Geometry: final body of the model. Coordinates: model frame, mm. A direction names the side the tool comes from. Give positions to 0.01 mm unless a question says otherwise; leave off trailing zeros. Write each loop counter-clockwise with the first axis right and the second up, starting at its lowest first coordinate (ties: lowest second). Pieces come first, ordered by that corner, then holes. Notation, with made-up numbers: (-5, 11) -> (43, 11) arc R8 cw to (43, 15) -> close; hole circle Ø6 at (-17.75, 3.25). An arc over 180 degrees is marked (long way). Answer as a JSON object with one key per item and string values.
from build123d import *

# Parameters (mm, degrees)
SKETCH_1_R        = 1
EXTRUDE_1_DEPTH   = 3
SKETCH_2_R        = 4.35
SKETCH_2_R_2      = 3.35
EXTRUDE_1_2_DEPTH = 3


with BuildPart() as part:
    # 草图1 → Extrude 1 (new body)
    with BuildSketch(Plane.XY):
        with BuildLine():
            Line((-2.463104237, 17.727922325), (-4.777267611, 4.407688076))
            ThreePointArc((-4.777267611, 4.407688076), (-6.49946928, 0.083060663), (-4.888346081, -4.284165332))
            Line((-4.888346081, -4.284165332), (-2.915337598, -17.659187952))
            ThreePointArc((-2.915337598, -17.659187952), (-0.505989798, -19.793533649), (2.009262058, -17.785077409))
            Line((2.009262058, -17.785077409), (4.663068788, -4.528331865))
            ThreePointArc((4.663068788, -4.528331865), (6.49946928, -0.083060663), (4.777267611, 4.407688076))
            Line((4.777267611, 4.407688076), (2.463104237, 17.727922325))
            ThreePointArc((2.463104237, 17.727922325), (0, 19.8), (-2.463104237, 17.727922325))
        make_face()
        with Locations((0, 7.5)):
            Circle(SKETCH_1_R, mode=Mode.SUBTRACT)
        with Locations((0, -7.5)):
            Circle(SKETCH_1_R, mode=Mode.SUBTRACT)
    extrude(amount=EXTRUDE_1_DEPTH)

    # 草图2 → Extrude 1 2 (add)
    with BuildSketch(Plane.XY.offset(3)):
        Circle(SKETCH_2_R)
        Circle(SKETCH_2_R_2, mode=Mode.SUBTRACT)
    extrude(amount=EXTRUDE_1_2_DEPTH)


solid = part.part
Q1. Set-up query: faces 4 (the cylindrical face through (-0.555, -19.792, 1.479)), 5 (the cylindrical face through (-3.347, 0.147, 4.479)). Return all of +Z, -Z, +X, -X, +Y, -Y with unobstructed straight access to the full face (end or side cutting, diameter ignored); none if empty.
Values:
{"face 4": "+Z, -Z, -Y", "face 5": "+Z"}
Q2. Cut plane A-A (z = 0.9). Return the cut outline in (x, y), and give its area (3 significant figures).
Values:
{"outline": "(-4.89, -4.28) -> (-2.92, -17.66) arc R2.5 ccw to (2.01, -17.79) -> (4.66, -4.53) arc R6.5 ccw to (4.78, 4.41) -> (2.46, 17.73) arc R2.5 ccw to (-2.46, 17.73) -> (-4.78, 4.41) arc R6.5 ccw to start; hole circle Ø2 at (0, -7.5); hole circle Ø2 at (0, 7.5)", "area": "307 mm²"}
Q3. Cut plane B-B (y = 7.5). Return the cut outline in (x, z), and give its area (3 significant figures).
Values:
{"outline": "(-4.24, 0) -> (-1, 0) -> (-1, 3) -> (-4.24, 3) -> close; (1, 0) -> (4.24, 0) -> (4.24, 3) -> (1, 3) -> close", "area": "19.4 mm²"}
Q4. Cut plane C-C (z = 3.9). Return the cut outline in (x, y), and give its area (3 significant figures).
Values:
{"outline": "circle Ø8.7 at (0, 0); hole circle Ø6.7 at (0, 0)", "area": "24.2 mm²"}
Q5. Material intervals for L1, parallel to Y at x = 0, z = 5; L2, parallel to Y at x = 0, z = 0.9; L3, parallel to Y at x = -0.5, z = 2, sorted ascending. Write a range as from..to.
Values:
{"L1": "-4.35..-3.35, 3.35..4.35", "L2": "-19.75..-8.5, -6.5..6.5, 8.5..19.8", "L3": "-19.79..-8.37, -6.63..6.63, 8.37..19.75"}
Q6. First-contact query: P1, Ø3.5, axis at x = -0.5, y = -1, coming from the +Z side; P2, Ø1.5, axis at x = 2.5, z = 3.5, coming from the +Y side. Flat tips, straight axial feed; report the tip coordinate or a pass-through.
Values:
{"P1": "z = 3", "P2": "y = 18.88"}
Q7. Mould query, pull axis Y, two halves, no side actions, for faces 1 (the cylindrical face through (-0.943, -4.247, 4.479)), 2 (the cylindrical face through (-0.13, -6.51, 1.48)), 3 (the flat face through (2, -3, 6)). Classes: pulls with the +Y half, pulls with the -Y half, needs draft (parallel to the pull), parting line crosses it, or undercut.
Values:
{"face 1": "parting line crosses it", "face 2": "undercut", "face 3": "needs draft"}
Q8. Cut plane D-D (x = 0). Return the cut outline in (y, z).
Values:
{"outline": "(-19.75, 0) -> (-8.5, 0) -> (-8.5, 3) -> (-19.75, 3) -> close; (-6.5, 0) -> (6.5, 0) -> (6.5, 3) -> (4.35, 3) -> (4.35, 6) -> (3.35, 6) -> (3.35, 3) -> (-3.35, 3) -> (-3.35, 6) -> (-4.35, 6) -> (-4.35, 3) -> (-6.5, 3) -> close; (8.5, 0) -> (19.8, 0) -> (19.8, 3) -> (8.5, 3) -> close"}
